```python
from build123d import *

# Parameters (mm, degrees)
EXTRUDE_THIN1_DEPTH = 350
SKETCH2_R           = 5
CUT_EXTRUDE1_DEPTH  = 623.208968113
FILLET1_R           = 10


with BuildPart() as part:
    # Sketch1 → Extrude-Thin1 (new, symmetric)
    with BuildSketch(Plane.XY):
        Polygon((-250, 50), (-250, 0), (250, 0), (250, 50), (256, 50), (256, -6), (-256, -6), (-256, 50), align=None)
    extrude(amount=EXTRUDE_THIN1_DEPTH, both=True)

    # Sketch2 → Cut-Extrude1 (cut, through all)
    with BuildSketch(Plane(origin=(256, 0, 0), x_dir=(0, 0, -1), z_dir=(1, 0, 0))):
        with Locations((320, 24)):
            Circle(SKETCH2_R)
        with BuildLine():
            Line((-300, 29), (0, 29))
            ThreePointArc((0, 29), (5, 24), (0, 19))
            Line((0, 19), (-300, 19))
            ThreePointArc((-300, 19), (-305, 24), (-300, 29))
        make_face()
    extrude(amount=-CUT_EXTRUDE1_DEPTH, mode=Mode.SUBTRACT)

    # Fillet1
    fillet1_edges = [part.edges().sort_by_distance(p)[0] for p in [
        (-253, 50, 350),
        (253, 50, 350),
        (-253, 50, -350),
        (253, 50, -350),
    ]]
    fillet(fillet1_edges, radius=FILLET1_R)


solid = part.part
```
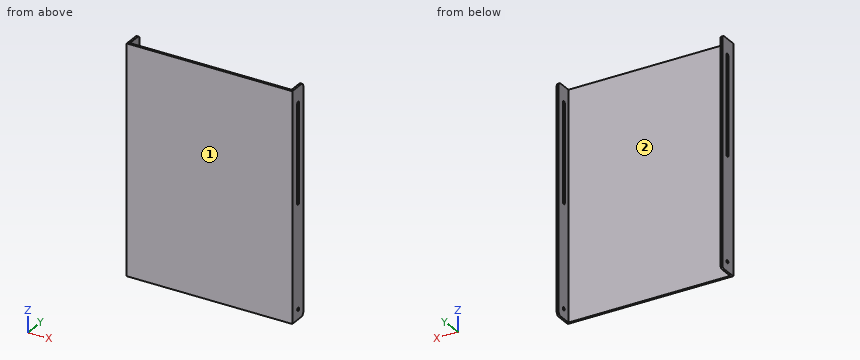
The listing builds one solid part. Answer for the finished solid, in the listing's coordinates (mm). Face numbers are marked on the shaded views. Give positions to 0.01 mm unless a question says otherwise; leave off trailing zeros. Loops run counter-clockwise (first coordinate to the right, second up) from the corner with the lowest first, then second, coordinate; pieces in that order, holes last. Notation, with made-up numbers: M -28.5,-8.5 L 14.5,-8.5 A17 cw 14.5,13.5 Z; hole C 47,-36 d9. An arc over 180 degrees is marked long. One line per item, written item: value.
Q1. Flat-ended cylindrical pins translate along their axes: P1, Ø8, axis at x = 194.5, y = 3.5, coming from the +Z side; P2, Ø6, axis at y = 24, z = -320, coming from the +X side; P3, Ø10, axis at x = 23.5, z = -63.5, coming from the +Y side. Find the tip coordinate at first contact, or state that the pin passes through.
Working result:
P1: stops at z = 350
P2: passes through
P3: stops at y = 0
Q2. Determine the mould class of the marked faces 1 and 2 for opening direction X: +X half, -X half, draft (parallel to the pull), parting line (faces both ways), or undercut.
Working result:
face 1: draft
face 2: undercut
Q3. Find the intervals of material crossed by line 1 (X direction, y = 17, z = -302); line 2 (Y direction, x = 252.4, z = -320); line 3 (Y direction, x = 163.5, z = 261), in increasing order. Write a range as from..to.
Working result:
line 1: x = -256..-250, 250..256
line 2: y = -6..19, 29..50
line 3: y = -6..0
Q4. A cutting plane is placed at B-B on z = -232. Determine the outline of the cut face in (x, y).
Working result:
outline: M -256,-6 L 256,-6 L 256,50 L 250,50 L 250,0 L -250,0 L -250,50 L -256,50 Z
Q5. A cutting plane is placed at C-C on x = -143. Determine the outline of the cut face in (y, z).
Working result:
outline: M -6,-350 L 0,-350 L 0,350 L -6,350 Z
Q6. A cutting plane is placed at A-A on z = 259.5. Determine the outline of the cut face in (x, y).
Working result:
outline: M -256,-6 L 256,-6 L 256,19 L 250,19 L 250,0 L -250,0 L -250,19 L -256,19 Z; M -256,29 L -250,29 L -250,50 L -256,50 Z; M 250,29 L 256,29 L 256,50 L 250,50 Z
